from build123d import *

# Parameters (mm, degrees)
SKETCH1_W                               = 279.4
SKETCH1_H                               = 279.4
BOSS_EXTRUDE1_DEPTH                     = 4.7625
CBORE_FOR_M6_HEX_HEAD_BOLT1_D           = 6.6
CBORE_FOR_M6_HEX_HEAD_BOLT1_CBORE_D     = 14.55
CBORE_FOR_M6_HEX_HEAD_BOLT1_CBORE_DEPTH = 4.38


with BuildPart() as part:
    # Sketch1 → Boss-Extrude1 (new body)
    with BuildSketch(Plane(origin=(0, 0, 0), x_dir=(1, 0, 0), z_dir=(0, 1, 0))):
        Rectangle(SKETCH1_W, SKETCH1_H)
    extrude(amount=BOSS_EXTRUDE1_DEPTH)

    # CBORE for M6 Hex Head Bolt1 (through all)
    with Locations(Plane(origin=(0, 4.7625, 0), x_dir=(1, 0, 0), z_dir=(0, 1, 0))):
        with Locations((-47.792708387, 76.2), (42.882092114, 76.2), (-47.792708387, 114.3), (42.882092114, 114.3), (76.2, 0), (114.3, 0)):
            CounterBoreHole(CBORE_FOR_M6_HEX_HEAD_BOLT1_D / 2, CBORE_FOR_M6_HEX_HEAD_BOLT1_CBORE_D / 2, CBORE_FOR_M6_HEX_HEAD_BOLT1_CBORE_DEPTH)


solid = part.part
Source: CAD feature listing. Evaluate the final solid. Frame: model axes, mm. A direction names the side the tool comes from. Coordinates: 2 decimals unless noted, no trailing zeros. Return JSON: item names as keys, results as strings.
Q1. Mould query, pull axis X, two halves, no side actions, for faces 3 (the flat face through (79.33, 0.383, 1.51)), 4 (the flat face through (-2, 0, -2)). Classes: released by +X, released by -X, zero draft, split by the parting line, or undercut.
Results:
{"face 3": "undercut", "face 4": "zero draft"}
Q2. Contact query for flat-ended pins moving along their axis: P1, Ø4.5, axis at x = 43.5, z = -112, coming from the +Y side; P2, Ø5.5, axis at x = 42.88, z = -114.3, coming from the +Y side. Output: stop coordinate, or through.
Results:
{"P1": "y = 0.38", "P2": "through"}
Q3. Access query for faces 1 (the cylindrical face through (68.932, 2.603, -0.32)), 2 (the cylindrical face through (117.6, 0.2, -0.1)). Directions: +Z, -Z, +X, -X, +Y, -Y. A direction counts if a zero-diameter tool reaches every point of the face in a straight line with its end or side. Return the directions, or none.
Results:
{"face 1": "+Y", "face 2": "+Y, -Y"}
Q4. Section A-A, the plane z = 0. Give the number of separate pieces and of enclosed holes in the cut face, plus the area to 3 significant figures.
Results:
{"separate pieces": "3", "enclosed holes": "0", "area": "1,200 mm2"}
Q5. Material intervals for line 1 along X through (y, z) = (0.15, -114.3); line 2 along Z through (x, y) = (-50.5, 0.55); line 3 along Z through (x, y) = (49, 2), sorted ascending.
Results:
{"line 1": "-139.7 to -51.09, -44.49 to 39.58, 46.18 to 139.7", "line 2": "-139.7 to -121.05, -107.55 to -82.95, -69.45 to 139.7", "line 3": "-139.7 to -118.24, -110.36 to -80.14, -72.26 to 139.7"}
